from build123d import *

# Parameters (mm, degrees)
EXTRUDE_1_DEPTH = 1
EXTRUDE_2_DEPTH = 30


with BuildPart() as part:
    # 草图1 → 凸台-拉伸1 (new, symmetric)
    with BuildSketch(Plane(origin=(0, 0, 0), x_dir=(1, 0, 0), z_dir=(0, 1, 0))):
        Polygon((-55, 0), (-55, 40), (-35.329752572, 113.410362798), (35.329752572, 113.410362798), (55, 40), (55, 0), align=None)
    extrude(amount=EXTRUDE_1_DEPTH, both=True)

    # 草图2 → 凸台-拉伸2 (add)
    with BuildSketch(Plane.XZ.offset(1)):
        Polygon((-42.690598923, -8), (-43.845299462, -6), (-46.154700538, -6), (-47.309401077, -8), (-46.154700538, -10), (-43.845299462, -10), align=None)
        Polygon((-27.690598923, -107.410362798), (-28.845299462, -105.410362798), (-31.154700538, -105.410362798), (-32.309401077, -107.410362798), (-31.154700538, -109.410362798), (-28.845299462, -109.410362798), align=None)
        Polygon((28.845299462, -109.410362798), (27.690598923, -107.410362798), (28.845299462, -105.410362798), (31.154700538, -105.410362798), (32.309401077, -107.410362798), (31.154700538, -109.410362798), align=None)
        Polygon((43.845299462, -10), (42.690598923, -8), (43.845299462, -6), (46.154700538, -6), (47.309401077, -8), (46.154700538, -10), align=None)
    extrude(amount=EXTRUDE_2_DEPTH)


solid = part.part
Check sheet for the modelled part. Datum: model origin and axes. Units: mm. Give positions to 0.01 mm unless a question says otherwise; leave off trailing zeros. Write each loop counter-clockwise with the first axis right and the second up, starting at its lowest first coordinate (ties: lowest second). Pieces come first, ordered by that corner, then holes. Notation, with made-up numbers: (-10.75, 56) -> (16.25, 56) arc R9 cw to (16.25, 69) -> close; hole circle Ø5 at (-3, 4). An arc over 180 degrees is marked (long way). Use one line per item in the form item = value. Start each with the question number.
1. Section check B-B (z = -26). Record the cut outline in (x, y).
2. Section check C-C (x = -2.5). Record the cut outline in (y, z).
3. Thickness scan on line 1 along Y through (x, z) = (4, -16.5); line 2 along X through (y, z) = (-5.5, -109); line 3 along Z through (x, y) = (29, -29). Record the ranges inside material, lowest first. Write a range as from..to.
4. Go/stop test with flat-tipped pins: P1, Ø2.5, axis at x = 30, y = -23, coming from the -Z side; P2, Ø2.5, axis at x = 45, y = -8.5, coming from the -Z side; P3, Ø0.7, axis at x = -45, y = -11.5, coming from the +Z side. Record where each tip stops, or that it passes through.
5. Section check A-A (y = -11). Record the cut outline in (x, z), and give its area (3 significant figures).
Conclusion:
q1.outline = (-55, -1) -> (55, -1) -> (55, 1) -> (-55, 1) -> close
q2.outline = (-1, -113.41) -> (1, -113.41) -> (1, 0) -> (-1, 0) -> close
q3.line_1 = -1..1
q3.line_2 = -31.39..-28.61, 28.61..31.39
q3.line_3 = -109.41..-105.41
q4.P1 = -109.41
q4.P2 = -10
q4.P3 = -6
q5.outline = (-47.31, -8) -> (-46.15, -10) -> (-43.85, -10) -> (-42.69, -8) -> (-43.85, -6) -> (-46.15, -6) -> close; (-32.31, -107.41) -> (-31.15, -109.41) -> (-28.85, -109.41) -> (-27.69, -107.41) -> (-28.85, -105.41) -> (-31.15, -105.41) -> close; (27.69, -107.41) -> (28.85, -109.41) -> (31.15, -109.41) -> (32.31, -107.41) -> (31.15, -105.41) -> (28.85, -105.41) -> close; (42.69, -8) -> (43.85, -10) -> (46.15, -10) -> (47.31, -8) -> (46.15, -6) -> (43.85, -6) -> close
q5.area = 55.4 mm²
